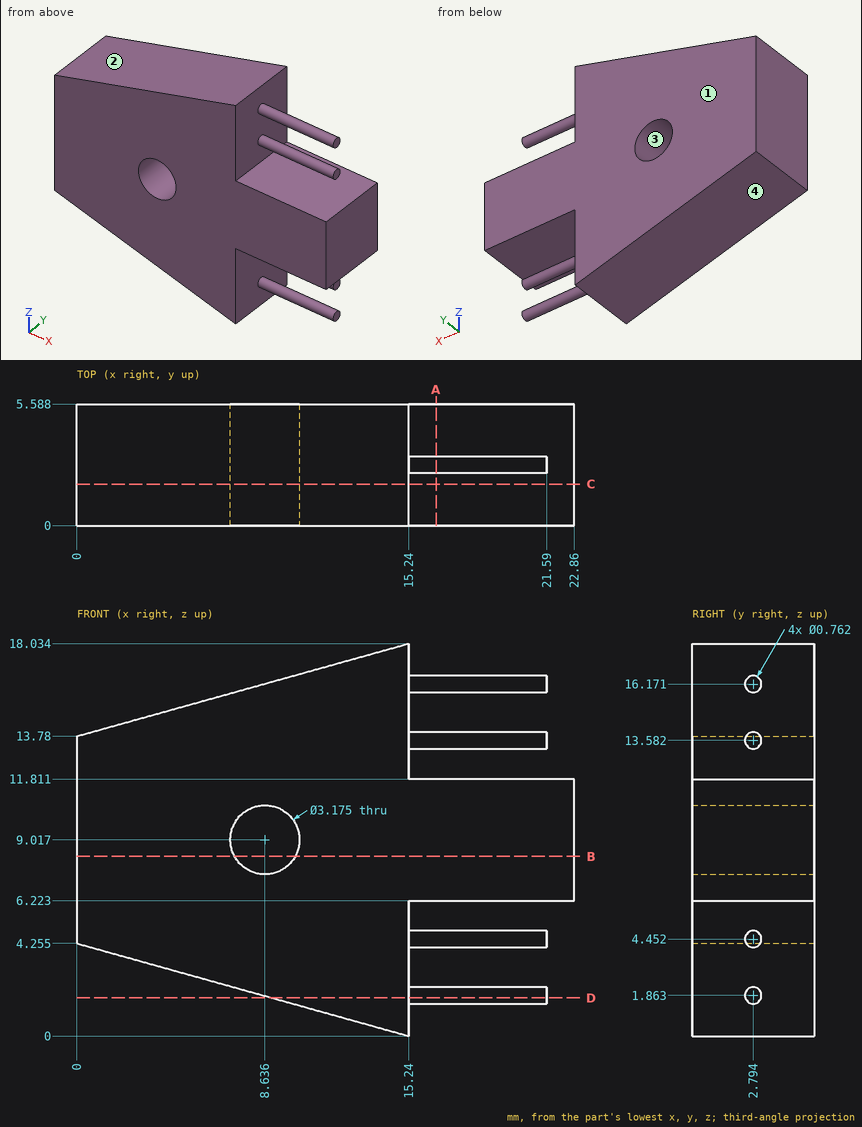
For this review, use the dimensioned drawing (mm, ordinates from the lowest corner) and the shaded views. Round coordinates to 2 decimals unless told otherwise and drop trailing zeros. Write each loop counter-clockwise with the first axis right and the second up, starting at its lowest first coordinate (ties: lowest second). Pieces come first, ordered by that corner, then holes. Notation, with made-up numbers: (61, 14) - (120, 14) arc R15 cw to (120, 22) - close; hole circle Ø7 at (-40, 16). An arc over 180 degrees is marked (long way). Answer as CSV lines item,"result". Start each with the question number.
(1) We need section A-A on x = 16.5. State the section outline as (y, z) points (1 decimal).
(2) For pin 1 Ø3 at (x, y) = (18.5, 4) entering from -Z; pin 2 Ø3 at (x, y) = (4, 3.5) entering from -Z; pin 3 Ø1.7 at (x, y) = (17.5, 3.5) entering from +Z, all flat-tipped, find the tip position at first contact; note any pin that passes through.
(3) To check wall thickness, follow line 1 (Z direction, x = 16.5, y = 2.5) (1 decimal); line 2 (Z direction, x = 16, y = 3.4); line 3 (X direction, y = 1.15, z = 5.5). State the ranges of each line that lie inside material, in increasing order.
(4) We need section B-B on z = 8.25. State the section outline as (x, y) points (1 decimal).
(5) We need section C-C on y = 1.9. State the section outline as (x, z) points (1 decimal), plus the area to 3 significant figures.
(6) Draft analysis for pull direction Z (two halves, no side actions). For the marked faces 1, 2, 3 and 4, state which applies: pulls with the +Z half, pulls with the -Z half, needs draft (parallel to the pull), parting line crosses it, or undercut.
(7) We need section D-D on z = 1.75. State the section outline as (x, y) points.
Worked answers:
1,outline,"(0, 6.2) - (5.6, 6.2) - (5.6, 11.8) - (0, 11.8) - close; circle Ø0.8 at (2.8, 1.9); circle Ø0.8 at (2.8, 4.5); circle Ø0.8 at (2.8, 13.6); circle Ø0.8 at (2.8, 16.2)"
2,pin 1,"z = 1.48"
2,pin 2,"z = 2.72"
2,pin 3,"z = 16.55"
3,line 1,"1.6 to 2.1, 4.2 to 4.7, 6.2 to 11.8, 13.3 to 13.8, 15.9 to 16.4"
3,line 2,"6.22 to 11.81"
3,line 3,"0 to 15.24"
4,outline,"(0, 0) - (7.2, 0) - (7.2, 5.6) - (0, 5.6) - close; (10, 0) - (22.9, 0) - (22.9, 5.6) - (10, 5.6) - close"
5,outline,"(0, 4.3) - (15.2, 0) - (15.2, 6.2) - (22.9, 6.2) - (22.9, 11.8) - (15.2, 11.8) - (15.2, 18) - (0, 13.8) - close; hole circle Ø3.2 at (8.6, 9)"
5,area,"245 mm²"
6,face 1,"needs draft"
6,face 2,"pulls with the +Z half"
6,face 3,"undercut"
6,face 4,"pulls with the -Z half"
7,outline,"(8.97, 0) - (15.24, 0) - (15.24, 2.43) - (21.59, 2.43) - (21.59, 3.16) - (15.24, 3.16) - (15.24, 5.59) - (8.97, 5.59) - close"
